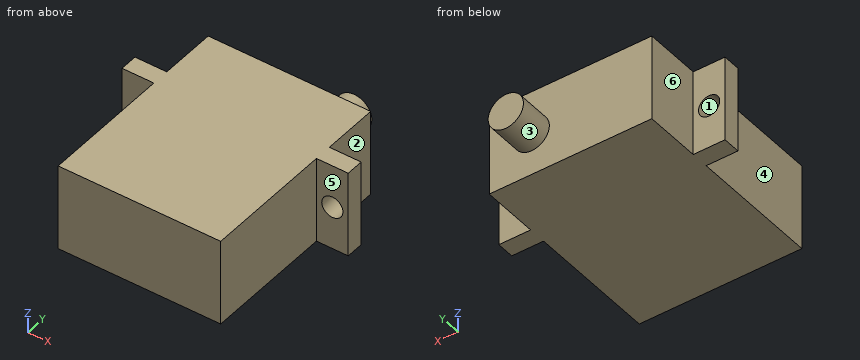
from build123d import *

# Parameters (mm, degrees)
SKETCH_1_W          = 23
SKETCH_1_H          = 12.2
EXTRUDE_1_DEPTH     = 29
SKETCH_2_W          = 32
SKETCH_2_H          = 2.5
EXTRUDE_2_DEPTH     = 12.2
SKETCH_3_R          = 1.5
CUT_EXTRUDE_1_DEPTH = 6
SKETCH_4_R          = 2.5
EXTRUDE_3_DEPTH     = 5


with BuildPart() as part:
    # Эскиз1 → Бобышка-Вытянуть1 (new body)
    with BuildSketch(Plane(origin=(0, 0, 0), x_dir=(1, 0, 0), z_dir=(0, 1, 0))):
        Rectangle(SKETCH_1_W, SKETCH_1_H)
    extrude(amount=EXTRUDE_1_DEPTH)

    # Эскиз2 → Бобышка-Вытянуть2 (add)
    with BuildSketch(Plane(origin=(0, 0, -6.1), x_dir=(-1, 0, 0), z_dir=(0, 0, -1))):
        with Locations((0, 19.75)):
            Rectangle(SKETCH_2_W, SKETCH_2_H)
    extrude(amount=-EXTRUDE_2_DEPTH)

    # Эскиз3 → Вырез-Вытянуть1 (cut)
    with BuildSketch(Plane(origin=(0, 21, 0), x_dir=(1, 0, 0), z_dir=(0, 1, 0))):
        with Locations(Location((13.75, 0, 0), (0, 0, 270))):
            Circle(SKETCH_3_R)
        with Locations(Location((-13.75, 0, 0), (0, 0, 90))):
            Circle(SKETCH_3_R)
    extrude(amount=-CUT_EXTRUDE_1_DEPTH, mode=Mode.SUBTRACT)

    # Эскиз4 → Бобышка-Вытянуть3 (add)
    with BuildSketch(Plane(origin=(0, 29, 0), x_dir=(1, 0, 0), z_dir=(0, 1, 0))):
        with Locations(Location((5.5, 0.1, 0), (0, 0, 90))):
            Circle(SKETCH_4_R)
    extrude(amount=EXTRUDE_3_DEPTH)


solid = part.part
The listing builds one solid part. Answer for the finished solid, in the listing's coordinates (mm). Face numbers are marked on the shaded views. A direction names the side the tool comes from. Round coordinates to 2 decimals unless told otherwise and drop trailing zeros. Order: outer loops, then holes, each group sorted by start corner. A loop starts at its lowest first (then second) coordinate and runs counter-clockwise, first axis right, second up. Notation, with made-up numbers: (45, 48.25) - (77, 48.25) arc R17 cw to (77, 61.25) - close; hole circle Ø11 at (25.5, 14.5). An arc over 180 degrees is marked (long way). Write item = value, one per line. Start each with the question number.
1) For a pull along Z with two mould halves and no side action, classify the marked faces 1, 2 and 3 as released by +Z, released by -Z, zero draft, split by the parting line, or undercut.
2) For the marked faces 4, 5 and 6, determine the directions among +Z, -Z, +X, -X, +Y, -Y from which every point of the face is accessible in a straight line to the end or side of a thin tool.
3) Section A-A, the plane x = -13.75 is taken. Write down the section's boundary in (y, z).
4) Section C-C, the plane x = 5.5 is taken. Write down the section's boundary in (y, z).
5) Straight lines are drawn through the part: L1, parallel to X at y = 20.4, z = 0; L2, parallel to Z at x = -13.75, y = 20.45; L3, parallel to Y at x = 2.5, z = -2.25. For each, find the intervals that lie inside material, in ascending order.
6) Section B-B, the plane z = 0 is taken. Write down the section's boundary in (x, y), plus the area to 3 significant figures.
7) Given pin 1 (3.5 mm diameter, centred on x = 13, z = 0.5, fed in from +Y); pin 2 (4 mm diameter, centred on y = 4, z = -4, fed in from +X); pin 3 (6 mm diameter, centred on y = 5.5, z = -2, fed in from -X), each flat-ended and moving along its own axis, determine where each tip first touches the part or whether it passes through.
8) Section D-D, the plane y = 20.5 is taken. Write down the section's boundary in (x, z), plus the area to 3 significant figures.
Results list:
q1.face_1 = undercut
q1.face_2 = zero draft
q1.face_3 = split by the parting line
q2.face_4 = +Z, -Z, -X, -Y
q2.face_5 = +Z, -Z, +X, -Y
q2.face_6 = +Z, -Z, -X, +Y
q3.outline = (18.5, -6.1) - (21, -6.1) - (21, -1.5) - (18.5, -1.5) - close; (18.5, 1.5) - (21, 1.5) - (21, 6.1) - (18.5, 6.1) - close
q4.outline = (0, -6.1) - (29, -6.1) - (29, -2.6) - (34, -2.6) - (34, 2.4) - (29, 2.4) - (29, 6.1) - (0, 6.1) - close
q5.L1 = -16 to -15.25, -12.25 to 12.25, 15.25 to 16
q5.L2 = -6.1 to -1.5, 1.5 to 6.1
q5.L3 = 0 to 29
q6.outline = (-16, 18.5) - (-15.25, 18.5) - (-15.25, 21) - (-16, 21) - close; (-12.25, 18.5) - (-11.5, 18.5) - (-11.5, 0) - (11.5, 0) - (11.5, 18.5) - (12.25, 18.5) - (12.25, 21) - (11.5, 21) - (11.5, 29) - (8, 29) - (8, 34) - (3, 34) - (3, 29) - (-11.5, 29) - (-11.5, 21) - (-12.25, 21) - close; (15.25, 18.5) - (16, 18.5) - (16, 21) - (15.25, 21) - close
q6.area = 699 mm^2
q7.pin_1 = 29
q7.pin_2 = 11.5
q7.pin_3 = -11.5
q8.outline = (-16, -6.1) - (16, -6.1) - (16, 6.1) - (-16, 6.1) - close; hole circle Ø3 at (-13.75, 0); hole circle Ø3 at (13.75, 0)
q8.area = 376 mm^2
